from build123d import *

# Parameters (mm, degrees)
EXTRUDE_1_DEPTH     = 3
SKETCH_2_R          = 1.5
CUT_EXTRUDE_1_DEPTH = 3


with BuildPart() as part:
    # 草图1 → 凸台-拉伸1 (new body)
    with BuildSketch(Plane.XY):
        with BuildLine():
            Line((0, 0), (15, 0))
            Line((15, 0), (29.498535682, -19.055218325))
            ThreePointArc((29.498535682, -19.055218325), (33.015661922, -21.959692608), (37.456822623, -23))
            Line((37.456822623, -23), (40, -23))
            ThreePointArc((40, -23), (43.535533906, -21.535533906), (45, -18))
            Line((45, -18), (45, -3))
            Line((45, -3), (60, -3))
            Line((60, -3), (60, -38))
            Line((60, -38), (-17.5, -38))
            Line((-17.5, -38), (-17.5, -23))
            Line((-17.5, -23), (0, 0))
        make_face()
    extrude(amount=EXTRUDE_1_DEPTH)

    # 草图2 → 切除-拉伸1 (cut)
    with BuildSketch(Plane.XY.offset(3)):
        with Locations((-13.5, -30.5)):
            Circle(SKETCH_2_R)
        with Locations((28.5, -30.5)):
            Circle(SKETCH_2_R)
        with Locations((7.5, -4)):
            Circle(SKETCH_2_R)
        with Locations((7.5, -17)):
            Circle(SKETCH_2_R)
        with Locations((52.5, -16)):
            Circle(SKETCH_2_R)
    extrude(amount=-CUT_EXTRUDE_1_DEPTH, mode=Mode.SUBTRACT)


solid = part.part
Input: part model. Units: mm. Frame: model coordinates. A direction names the side the tool comes from. Coordinates: 2 decimals unless noted, no trailing zeros. Loops run counter-clockwise (first coordinate to the right, second up) from the corner with the lowest first, then second, coordinate; pieces in that order, holes last. Notation, with made-up numbers: (0.5, 6) - (35.5, 6) arc R19 ccw to (35.5, 34) - close; hole circle Ø11 at (70.25, 1). An arc over 180 degrees is marked (long way). Answer in a Markdown table with one row per item. Add a question column.
Item 1: Access query for faces 1 (the flat face through (52, -3, 1)), 2 (the flat face through (60, -20, 1)), 3 (the flat face through (22.148, -9.394, 1.479)). Directions: +Z, -Z, +X, -X, +Y, -Y. A direction counts if a zero-diameter tool reaches every point of the face in a straight line with its end or side. Return the directions, or none.
Item 2: Section query A-A on z = 1.35. Return the cut outline in (x, y).
Item 3: Mould query, pull axis Y, two halves, no side actions, for faces 4 (the cylindrical face through (6.39, -15.99, 1.52)), 5 (the flat face through (22, -23, 3)), 6 (the flat face through (-8.9, -11.7, 1.5)). Classes: released by +Y, released by -Y, zero draft, split by the parting line, or undercut.
Item 4: Section query B-B on y = -11. Return the cut outline in (x, z).
Item 5: Contact query for flat-ended pins moving along their axis: P1, Ø2.5, axis at x = 52.5, y = -16, coming from the +Z side; P2, Ø1.3, axis at x = 39, z = 1, coming from the +Y side. Output: stop coordinate, or through.
Item 6: Line query: line 1 along Y through (x, z) = (7.5, 2.15); line 2 along Y through (x, z) = (52.5, 1.5); line 3 along X through (y, z) = (-4.5, 1.2). Output: solid intervals per line, ascending. Write a range as [from, to].
Item 7: Section query C-C on x = 28.5. Return the cut outline in (y, z), then the cut area to 3 significant figures.
Item 8: Section query D-D on y = -4. Return the cut outline in (x, z), then the cut area to 3 significant figures.
Recorded:
| question | item | result |
|---|---|---|
| 1 | face 1 | +Z, -Z, +X, +Y |
| 1 | face 2 | +Z, -Z, +X, +Y, -Y |
| 1 | face 3 | +Z, -Z, +Y |
| 2 | outline | (-17.5, -38) - (60, -38) - (60, -3) - (45, -3) - (45, -18) arc R5 cw to (40, -23) - (37.46, -23) arc R10 cw to (29.5, -19.06) - (15, 0) - (0, 0) - (-17.5, -23) - close; hole circle Ø3 at (-13.5, -30.5); hole circle Ø3 at (7.5, -17); hole circle Ø3 at (7.5, -4); hole circle Ø3 at (28.5, -30.5); hole circle Ø3 at (52.5, -16) |
| 3 | face 4 | undercut |
| 3 | face 5 | zero draft |
| 3 | face 6 | released by +Y |
| 4 | outline | (-8.37, 0) - (23.37, 0) - (23.37, 3) - (-8.37, 3) - close; (45, 0) - (60, 0) - (60, 3) - (45, 3) - close |
| 5 | P1 | through |
| 5 | P2 | y = -23 |
| 6 | line 1 | [-38, -18.5], [-15.5, -5.5], [-2.5, 0] |
| 6 | line 2 | [-38, -17.5], [-14.5, -3] |
| 6 | line 3 | [-3.42, 6.09], [8.91, 18.42], [45, 60] |
| 7 | outline | (-38, 0) - (-32, 0) - (-32, 3) - (-38, 3) - close; (-29, 0) - (-17.74, 0) - (-17.74, 3) - (-29, 3) - close |
| 7 | area | 51.8 mm^2 |
| 8 | outline | (-3.04, 0) - (6, 0) - (6, 3) - (-3.04, 3) - close; (9, 0) - (18.04, 0) - (18.04, 3) - (9, 3) - close; (45, 0) - (60, 0) - (60, 3) - (45, 3) - close |
| 8 | area | 99.3 mm^2 |
